Drawing for the job (mm, zero at the part's lowest x, y, z). A direction names the side the tool comes from. Give positions to 0.01 mm unless a question says otherwise; leave off trailing zeros. Order: outer loops, then holes, each group sorted by start corner. A loop starts at its lowest first (then second) coordinate and runs counter-clockwise, first axis right, second up. Notation, with made-up numbers: (57, 18) - (78, 18) arc R15 ccw to (78, 24) - close; hole circle Ø11 at (62.25, 39). An arc over 180 degrees is marked (long way). Use a Markdown table: item, result. Add a question column.
(1) Slice it at A-A (y = 117.5). Write the cut outline in (x, z) (1 decimal).
(2) Slice it at C-C (z = 34). Write the cut outline in (x, y).
(3) Flat gauge pins, fed straight in: pin 1 (1.5 mm diameter, centred on y = 98.5, z = 36.5, fed in from -X) (1 decimal); pin 2 (15 mm diameter, centred on x = 672.5, z = 28, fed in from +Y); pin 3 (6 mm diameter, centred on x = 553, z = 35.5, fed in from +Y). Where does each tip first touch, or does it go through?
(4) Which spindle directions (+Z, -Z, +X, -X, +Y, -Y) get a long thin tool onto all of the face, cutting with end or side? Do the marked faces 1, 2, 3, 4 and 5. Say none if no direction does.
(5) Slice it at D-D (y = 485.5). Write the cut outline in (x, z), then the cut area to 3 significant figures.
(6) Wall check: line 1 (Y direction, x = 349, z = 33.5) (1 decimal); line 2 (X direction, y = 346, z = 48); line 3 (Y direction, x = 380, z = 16.5). Give the ranges that are in metal, low to high.
(7) Slice it at B-B (x = 48.5). Write the cut outline in (y, z).
(8) Mould opens along Y. For the marked faces 6, 7, 8 and 9 say: +Y half, -Y half, draft (parallel to the pull), parting line (faces both ways), or undercut.
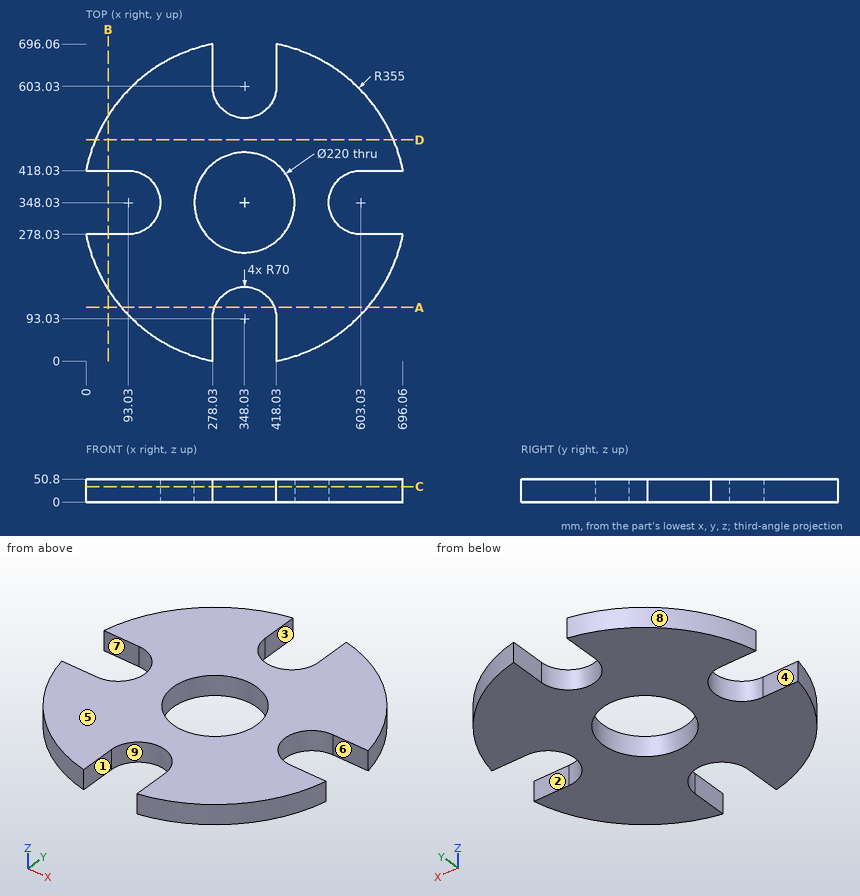
Solution:
| question | item | result |
|---|---|---|
| 1 | outline | (78.1, 0) - (282.4, 0) - (282.4, 50.8) - (78.1, 50.8) - close; (413.6, 0) - (618, 0) - (618, 50.8) - (413.6, 50.8) - close |
| 2 | outline | (0, 278.03) arc R355 ccw to (278.03, 0) - (278.03, 93.03) arc R70 cw to (418.03, 93.03) - (418.03, 0) arc R355 ccw to (696.06, 278.03) - (603.03, 278.03) arc R70 cw to (603.03, 418.03) - (696.06, 418.03) arc R355 ccw to (418.03, 696.06) - (418.03, 603.03) arc R70 cw to (278.03, 603.03) - (278.03, 696.06) arc R355 ccw to (0, 418.03) - (93.03, 418.03) arc R70 cw to (93.03, 278.03) - close; hole circle Ø220 at (348.03, 348.03) |
| 3 | pin 1 | x = 94.8 |
| 3 | pin 2 | y = 507.89 |
| 3 | pin 3 | y = 639.98 |
| 4 | face 1 | +Z, -Z, -Y |
| 4 | face 2 | +Z, -Z, +X |
| 4 | face 3 | +Z, -Z, +Y |
| 4 | face 4 | +Z, -Z, -X |
| 4 | face 5 | +Z, +X, -X, +Y, -Y |
| 5 | outline | (20.73, 0) - (675.33, 0) - (675.33, 50.8) - (20.73, 50.8) - close |
| 5 | area | 33,300 mm2 |
| 6 | line 1 | 163 to 238, 458 to 533 |
| 6 | line 2 | 163 to 238.05, 458.01 to 533.06 |
| 6 | line 3 | 155.3 to 242.78, 453.28 to 540.76 |
| 7 | outline | (157.49, 0) - (278.03, 0) - (278.03, 50.8) - (157.49, 50.8) - close; (418.03, 0) - (538.57, 0) - (538.57, 50.8) - (418.03, 50.8) - close |
| 8 | face 6 | undercut |
| 8 | face 7 | undercut |
| 8 | face 8 | +Y half |
| 8 | face 9 | -Y half |
